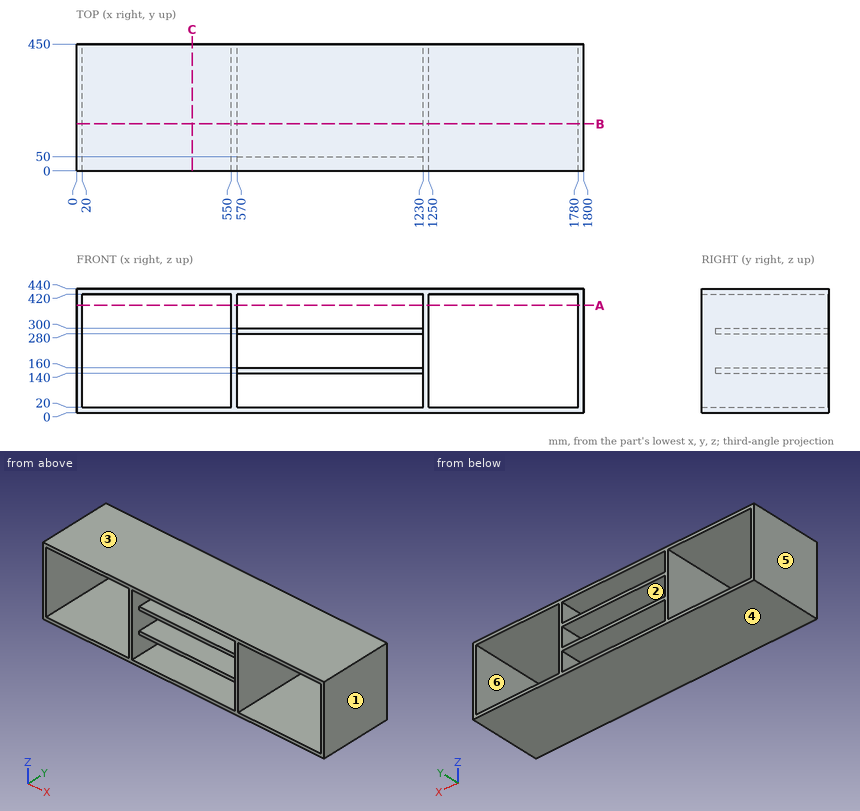
Drawing for the job (mm, zero at the part's lowest x, y, z). A direction names the side the tool comes from. Give positions to 0.01 mm unless a question says otherwise; leave off trailing zeros. Order: outer loops, then holes, each group sorted by start corner. A loop starts at its lowest first (then second) coordinate and runs counter-clockwise, first axis right, second up. Notation, with made-up numbers: M 82,85 L 92,85 A21 ccw 92,106 Z; hole C 43.5,-7.5 d9. An arc over 180 degrees is marked long. Put each result on its own line as item: value. Start each with the question number.
(1) Saw through at B-B, the plane y = 166.5. Write the cut outline in (x, z), then the cut area to 3 significant figures.
(2) Mould opens along Z. For the marked faces 1, 2, 3 and 4 say: +Z half, -Z half, draft (parallel to the pull), parting line (faces both ways), or undercut.
(3) Flat gauge pin, fed straight in: pin 1 Ø10 at (x, z) = (1028.5, 154) entering from -Y. Where does the tip first touch, or does it go through?
(4) Saw through at C-C, the plane x = 410. Write the cut outline in (y, z).
(5) Drill centre lines: line 1 along X through (y, z) = (423.5, 158); line 2 along X through (y, z) = (45, 414); line 3 along Z through (x, y) = (788, 113.5). Where is each one in solid material? Low to high.
(6) Which spindle directions (+Z, -Z, +X, -X, +Y, -Y) get a long thin tool onto all of the face, cutting with end or side? Do the marked faces 5 and 6. Say none if no direction does.
(7) Saw through at A-A, the plane z = 381. Write the cut outline in (x, y).
Check result:
1. outline: M 0,0 L 1800,0 L 1800,440 L 0,440 Z; hole M 20,20 L 550,20 L 550,420 L 20,420 Z; hole M 570,20 L 1230,20 L 1230,140 L 570,140 Z; hole M 570,160 L 1230,160 L 1230,280 L 570,280 Z; hole M 570,300 L 1230,300 L 1230,420 L 570,420 Z; hole M 1250,20 L 1780,20 L 1780,420 L 1250,420 Z
1. area: 130,000 mm2
2. face 1: draft
2. face 2: undercut
2. face 3: +Z half
2. face 4: -Z half
3. pin 1: stops at y = 50
4. outline: M 0,0 L 450,0 L 450,20 L 0,20 Z; M 0,420 L 450,420 L 450,440 L 0,440 Z
5. line 1: x = 0 to 20, 550 to 1250, 1780 to 1800
5. line 2: x = 0 to 20, 550 to 570, 1230 to 1250, 1780 to 1800
5. line 3: z = 0 to 20, 140 to 160, 280 to 300, 420 to 440
6. face 5: +Z, -Z, -X, +Y, -Y
6. face 6: +Y, -Y
7. outline: M 0,0 L 20,0 L 20,450 L 0,450 Z; M 550,0 L 570,0 L 570,450 L 550,450 Z; M 1230,0 L 1250,0 L 1250,450 L 1230,450 Z; M 1780,0 L 1800,0 L 1800,450 L 1780,450 Z
